from build123d import *

# Parameters (mm, degrees)
F1_DEPTH       = 30
F2_SIZE        = 5
F3_SIZE        = 1
F5_D           = 3
F5_CSINK_D     = 6
F5_CSINK_ANGLE = 90
F7_D           = 3
F7_CSINK_D     = 6
F7_CSINK_ANGLE = 90


with BuildPart() as f1:
    # F0 (on Right) → F1 (new body)
    with BuildSketch(Plane.YZ):
        Polygon((-25, 0), (0, 0), (0, 25), (-3, 25), (-3, 3), (-25, 3), align=None)
    extrude(amount=F1_DEPTH)

    # F2
    f2_edges = [f1.edges().sort_by_distance(p)[0] for p in [
        (15, -3, 3),
    ]]
    chamfer(f2_edges, length=F2_SIZE)

    # F3
    f3_edges = [f1.edges().sort_by_distance(p)[0] for p in [
        (15, 0, 0),
    ]]
    chamfer(f3_edges, length=F3_SIZE)

    # F5 (through all)
    with Locations(Plane.XZ.offset(3)):
        with Locations((15, 17)):
            CounterSinkHole(F5_D / 2, F5_CSINK_D / 2, counter_sink_angle=F5_CSINK_ANGLE)

    # F7 (through all)
    with Locations(Plane.XY.offset(3)):
        with Locations((15, -17)):
            CounterSinkHole(F7_D / 2, F7_CSINK_D / 2, counter_sink_angle=F7_CSINK_ANGLE)


solid = f1.part
Verification items for the finished model (mm, model axes). A direction names the side the tool comes from. Coordinates: 2 decimals unless noted, no trailing zeros. Order: outer loops, then holes, each group sorted by start corner. A loop starts at its lowest first (then second) coordinate and runs counter-clockwise, first axis right, second up. Notation, with made-up numbers: (80, -24.75) -> (112, -24.75) arc R26 cw to (112, 12.25) -> close; hole circle Ø2 at (-27, 17). An arc over 180 degrees is marked (long way). Use CSV: the item, a comma, the result in double quotes. Start each with the question number.
Q1. Section check A-A, the plane z = 17. Record the cut outline in (x, y), and give its area (4 significant figures).
Q2. Draft check along Z on faces 1 (the flat face through (15, -1, 25)), 2 (the flat face through (14.8, -0.5, 0.5)), 3 (the conical face through (17, -2, 17)), 4 (the flat face through (30, -5, 5)). Enter one of: +Z half, -Z half, draft (parallel to the pull), parting line (faces both ways), or undercut.
Q3. Tool access check on faces 5 (the flat face through (11, -3, 17)), 6 (the flat face through (15, 0, 13)). Record the directions out of +Z, -Z, +X, -X, +Y, -Y that give a thin tool (end or side, any length) a straight path to the whole face; none if there is none.
Q4. Section check B-B, the plane x = 15. Record the cut outline in (y, z), and give its area (4 significant figures).
Q5. Depth check by flat-ended pin: P1, Ø13.5, axis at x = 13, y = -12.5, coming from the +Z side; P2, Ø5, axis at x = 11, z = 18, coming from the -Y side; P3, Ø4, axis at x = 15, z = 17, coming from the -Y side. Enter the tip coordinate at first touch or a pass-through.
Q6. Thickness scan on line 1 along X through (y, z) = (-17, 0.4); line 2 along Y through (x, z) = (17.25, 20.25); line 3 along Z through (x, y) = (9.25, -22.5). Record the ranges inside material, lowest first.
Q7. Section check D-D, the plane x = 19.25. Record the cut outline in (y, z).
Q8. Section check C-C, the plane y = -17. Record the cut outline in (x, z), and give its area (4 significant figures).
Returned:
1,outline,"(0, -3) -> (12, -3) -> (13.5, -1.5) -> (13.5, 0) -> (0, 0) -> close; (16.5, -1.5) -> (18, -3) -> (30, -3) -> (30, 0) -> (16.5, 0) -> close"
1,area,"78.75 mm^2"
2,face 1,"+Z half"
2,face 2,"-Z half"
2,face 3,"undercut"
2,face 4,"draft"
3,face 5,"+Z, +X, -X, -Y"
3,face 6,"+Z, -Z, +X, -X, +Y"
4,outline,"(-25, 0) -> (-18.5, 0) -> (-18.5, 1.5) -> (-20, 3) -> (-25, 3) -> close; (-15.5, 0) -> (-1, 0) -> (0, 1) -> (0, 15.5) -> (-1.5, 15.5) -> (-3, 14) -> (-3, 8) -> (-8, 3) -> (-14, 3) -> (-15.5, 1.5) -> close; (-3, 20) -> (-1.5, 18.5) -> (0, 18.5) -> (0, 25) -> (-3, 25) -> close"
4,area,"130.5 mm^2"
5,P1,"stops at z = 5.25"
5,P2,"stops at y = -3"
5,P3,"stops at y = -2"
6,line 1,"x = 0 to 13.5, 16.5 to 30"
6,line 2,"y = -3 to 0"
6,line 3,"z = 0 to 3"
7,outline,"(-25, 0) -> (-1, 0) -> (0, 1) -> (0, 25) -> (-3, 25) -> (-3, 8) -> (-8, 3) -> (-25, 3) -> close"
8,outline,"(0, 0) -> (13.5, 0) -> (13.5, 1.5) -> (12, 3) -> (0, 3) -> close; (16.5, 0) -> (30, 0) -> (30, 3) -> (18, 3) -> (16.5, 1.5) -> close"
8,area,"78.75 mm^2"
